Input: dimensioned drawing with shaded views. Units: mm. Origin: part minimum x, y, z. A direction names the side the tool comes from. Give positions to 0.01 mm unless a question says otherwise; leave off trailing zeros. Order: outer loops, then holes, each group sorted by start corner. A loop starts at its lowest first (then second) coordinate and runs counter-clockwise, first axis right, second up.
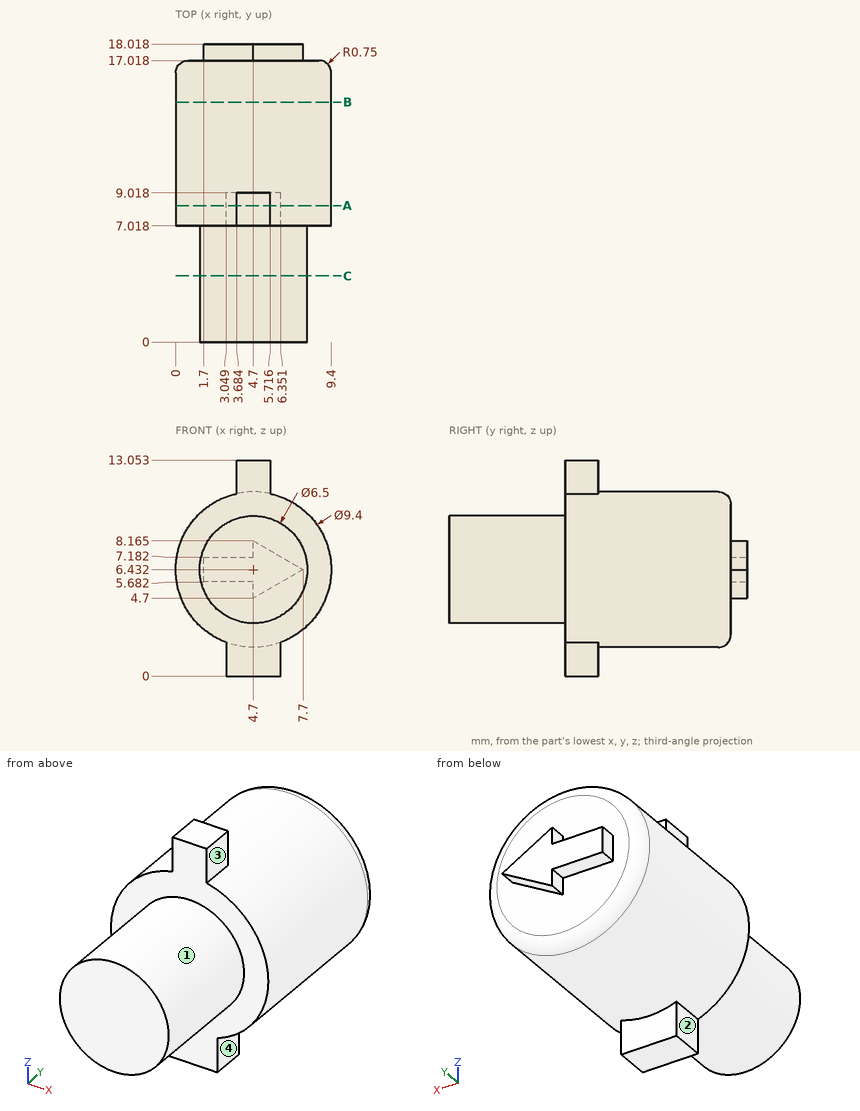
1) Reachability of the marked faces 1, 2, 3 and 4 from +Z, -Z, +X, -X, +Y, -Y: full face, straight path, thin tool, end or side. Return the list, or none.
Report:
face 1: -Y
face 2: -Z, -X, +Y, -Y
face 3: +Z, +X, +Y, -Y
face 4: -Z, +X, +Y, -Y
2) Pin query (flat end, axial travel): pin 1 (3 mm diameter, centred on y = 6.5, z = 3.5, fed in from -X) (1 decimal); pin 2 (0.6 mm diameter, centred on y = 8.5, z = 12.5, fed in from -X); pin 3 (0.5 mm diameter, centred on y = 17.5, z = 7.5, fed in from -X). Return the tip coordinate at first contact, or that it passes through.
Report:
pin 1: stops at x = 0.3
pin 2: stops at x = 3.68
pin 3: stops at x = 4.7
3) Material intervals for L1, parallel to Y at x = 2.5, z = 5; L2, parallel to Y at x = 4.5, z = 1; L3, parallel to X at y = 10.25, z = 6.25, sorted ascending.
Report:
L1: y = 0 to 17.02
L2: y = 7.02 to 9.02
L3: x = 0 to 9.4
4) Section query A-A, the plane y = 8.25. Return the cut outline in (x, z).
Report:
outline: (3.05, 0) - (6.35, 0) - (6.35, 2.03) arc R4.7 ccw to (5.72, 11.02) - (5.72, 13.05) - (3.68, 13.05) - (3.68, 11.02) arc R4.7 ccw to (3.05, 2.03) - close
5) Section query B-B, the plane y = 14.5. Return the cut outline in (x, z).
Report:
outline: circle Ø9.4 at (4.7, 6.43)
6) Section query C-C, the plane y = 4. Return the cut outline in (x, z), and give its area (3 significant figures).
Report:
outline: circle Ø6.5 at (4.7, 6.43)
area: 33.2 mm2
